Source: three-view drawing plus pictorial views. Frame: mm from the lowest corner of the part. Give positions to 0.01 mm unless a question says otherwise; leave off trailing zeros. Loops run counter-clockwise (first coordinate to the right, second up) from the corner with the lowest first, then second, coordinate; pieces in that order, holes last.
1. Material intervals for line 1 along Y through (x, z) = (70, 0.55) (1 decimal); line 2 along Y through (x, z) = (106.5, 0.75) (1 decimal); line 3 along X through (y, z) = (152, 0.8) (1 decimal), sorted ascending.
2. Section A-A, the plane x = 103.5. Output: boundary loops of the cut face in (y, z) (1 decimal), then the cut area to 3 significant figures.
3. Section C-C, the plane z = 1.95. State how many separate pieces and enclosed holes the cut face has, then the cut area to 3 significant figures.
4. First-contact query: P1, Ø1.6, axis at y = 31, z = 2, coming from the -X side; P2, Ø1, axis at y = 150.5, z = 1, coming from the +X side. Flat tips, straight axial feed; report the tip coordinate or a pass-through.
5. Section B-B, the plane y = 98. Output: boundary loops of the cut face in (x, z) (1 decimal).
6. Section D-D, the plane x = 48.5. Output: boundary loops of the cut face in (y, z) (1 decimal).
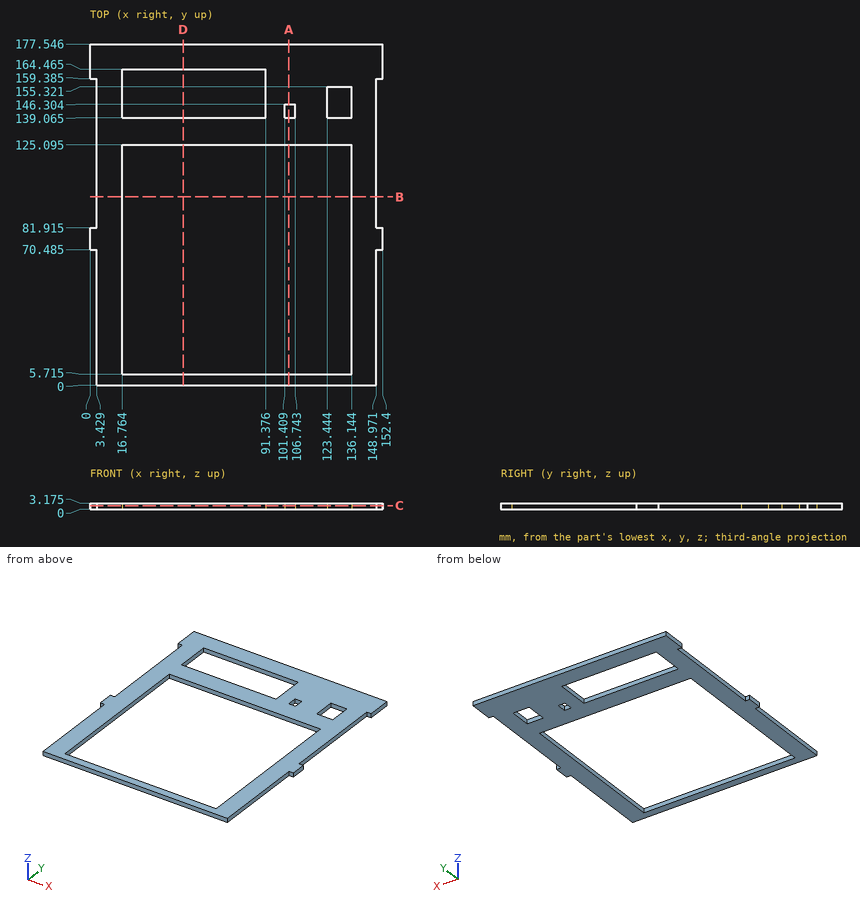
Answers below:
1. line 1: y = 0 to 5.7, 125.1 to 139.1, 164.5 to 177.5
1. line 2: y = 0 to 5.7, 125.1 to 139.1, 146.3 to 177.5
1. line 3: x = 3.4 to 16.8, 91.4 to 123.4, 136.1 to 149
2. outline: (0, 0) - (5.7, 0) - (5.7, 3.2) - (0, 3.2) - close; (125.1, 0) - (139.1, 0) - (139.1, 3.2) - (125.1, 3.2) - close; (146.3, 0) - (177.5, 0) - (177.5, 3.2) - (146.3, 3.2) - close
2. area: 162 mm2
3. separate pieces: 1
3. enclosed holes: 4
3. area: 9,650 mm2
4. P1: stops at x = 3.43
4. P2: stops at x = 148.97
5. outline: (3.4, 0) - (16.8, 0) - (16.8, 3.2) - (3.4, 3.2) - close; (136.1, 0) - (149, 0) - (149, 3.2) - (136.1, 3.2) - close
6. outline: (0, 0) - (5.7, 0) - (5.7, 3.2) - (0, 3.2) - close; (125.1, 0) - (139.1, 0) - (139.1, 3.2) - (125.1, 3.2) - close; (164.5, 0) - (177.5, 0) - (177.5, 3.2) - (164.5, 3.2) - close
